```python
from build123d import *

# Parameters (mm, degrees)
SKETCH5_W                 = 81.2
SKETCH5_H                 = 81.2
BOSS_EXTRUDE3_DEPTH       = 2
SKETCH9_W                 = 81.2
SKETCH9_H                 = 81.2
SKETCH9_W_2               = 75.5
SKETCH9_H_2               = 75.5
BOSS_EXTRUDE5_DEPTH       = 5
SKETCH6_W                 = 42.5
SKETCH6_H                 = 57.5
SKETCH6_W_2               = 38.5
SKETCH6_H_2               = 53.5
BOSS_EXTRUDE4_DEPTH       = 17.4
SKETCH7_W                 = 28.5
SKETCH7_H                 = 43.5
SKETCH7_W_2               = 27
SKETCH7_H_2               = 6
SKETCH7_W_3               = 53
CUT_EXTRUDE1_DEPTH        = 2
SKETCH10_W                = 6.5
SKETCH10_H                = 0.85
BOSS_EXTRUDE6_DEPTH       = 15
BOSS_EXTRUDE7_OUTLINE_W   = 81.2
BOSS_EXTRUDE7_OUTLINE_H   = 81.2
BOSS_EXTRUDE7_OUTLINE_W_2 = 79.2
BOSS_EXTRUDE7_OUTLINE_H_2 = 79.2
BOSS_EXTRUDE7_OUTLINE_W_3 = 77.5
BOSS_EXTRUDE7_OUTLINE_H_3 = 77.5
BOSS_EXTRUDE7_OUTLINE_W_4 = 75.5
BOSS_EXTRUDE7_OUTLINE_H_4 = 75.5
BOSS_EXTRUDE7_DEPTH       = 5


# Read off the part's stored shape, not the designer's step: Boss-Extrude7
with BuildPart() as part:
    # Sketch5 → Boss-Extrude3 (new body)
    with BuildSketch(Plane(origin=(0, 0, 0), x_dir=(1, 0, 0), z_dir=(0, 1, 0))):
        with Locations((39.6, 39.6)):
            Rectangle(SKETCH5_W, SKETCH5_H)
    extrude(amount=BOSS_EXTRUDE3_DEPTH)

    # Sketch9 → Boss-Extrude5 (add)
    with BuildSketch(Plane.XZ):
        with Locations((39.6, -39.6)):
            Rectangle(SKETCH9_W, SKETCH9_H)
        with Locations((39.6, -39.6)):
            Rectangle(SKETCH9_W_2, SKETCH9_H_2, mode=Mode.SUBTRACT)
    extrude(amount=BOSS_EXTRUDE5_DEPTH)

    # Sketch6 → Boss-Extrude4 (add)
    with BuildSketch(Plane.XZ):
        with Locations((52.1, -39.6)):
            Rectangle(SKETCH6_W, SKETCH6_H)
        with Locations((52.1, -39.6)):
            Rectangle(SKETCH6_W_2, SKETCH6_H_2, mode=Mode.SUBTRACT)
    extrude(amount=BOSS_EXTRUDE4_DEPTH)

    # Sketch7 → Cut-Extrude1 (cut)
    with BuildSketch(Plane.XZ):
        with Locations((52.1, -39.6)):
            Rectangle(SKETCH7_W, SKETCH7_H)
        with Locations((63.85, -5.85)):
            Rectangle(SKETCH7_W_2, SKETCH7_H_2)
        with Locations((50.85, -73.35)):
            Rectangle(SKETCH7_W_3, SKETCH7_H_2)
    extrude(amount=-CUT_EXTRUDE1_DEPTH, mode=Mode.SUBTRACT)

    # Sketch10 → Boss-Extrude6 (add)
    with BuildSketch(Plane.XZ.offset(5)):
        with Locations((24.5, -0.425)):
            Rectangle(SKETCH10_W, SKETCH10_H)
    extrude(amount=BOSS_EXTRUDE6_DEPTH)

    # Boss-Extrude7 outline → Boss-Extrude7 (add)
    # profile 1 of 2: a face of its own
    with BuildSketch(Plane(origin=(0, -5, 0), x_dir=(-1, 0, 0), z_dir=(0, -1, 0))):
        with Locations((-39.6, 39.6)):
            Rectangle(BOSS_EXTRUDE7_OUTLINE_W, BOSS_EXTRUDE7_OUTLINE_H)
        with Locations((-39.6, 39.6)):
            Rectangle(BOSS_EXTRUDE7_OUTLINE_W_2, BOSS_EXTRUDE7_OUTLINE_H_2, mode=Mode.SUBTRACT)
    # profile 2 of 2: a face of its own
    with BuildSketch(Plane(origin=(0, -5, 0), x_dir=(-1, 0, 0), z_dir=(0, -1, 0))):
        with Locations((-39.6, 39.6)):
            Rectangle(BOSS_EXTRUDE7_OUTLINE_W_3, BOSS_EXTRUDE7_OUTLINE_H_3)
        with Locations((-39.6, 39.6)):
            Rectangle(BOSS_EXTRUDE7_OUTLINE_W_4, BOSS_EXTRUDE7_OUTLINE_H_4, mode=Mode.SUBTRACT)
    extrude(amount=BOSS_EXTRUDE7_DEPTH)


solid = part.part
```
Here's how the part is built. I have some questions about the finished solid (model axes, mm). A direction names the side the tool comes from. Give positions to 0.01 mm unless a question says otherwise; leave off trailing zeros. Write each loop counter-clockwise with the first axis right and the second up, starting at its lowest first coordinate (ties: lowest second). Pieces come first, ordered by that corner, then holes. Notation, with made-up numbers: (57, 0) -> (106, 0) arc R26 ccw to (106, 29) -> close; hole circle Ø1 at (85.25, 20). An arc over 180 degrees is marked (long way). Use one line per item in the form item = value.
1) If I drill on L1, parallel to X at y = -8, z = -65; L2, parallel to X at y = -8.5, z = -10; L3, parallel to Z at x = 67, y = 0.25, over which ranges is the centre line in solid material (lowest first)? Write a range as [from, to].
Verdict:
L1 = [-1, 0], [0.85, 1.85], [30.85, 32.85], [71.35, 73.35], [77.35, 78.35], [79.2, 80.2]
L2 = [-1, 0], [0.85, 1.85], [77.35, 78.35], [79.2, 80.2]
L3 = [-80.2, -76.35], [-70.35, -8.85], [-2.85, 1]
2) I'm going to push flat-ended pins straight in: pin 1 (8 mm diameter, centred on x = 61.5, z = -26, fed in from +Y); pin 2 (8 mm diameter, centred on x = 53, y = -15.5, fed in from +Z); pin 3 (12.5 mm diameter, centred on x = 62, z = -47.5, fed in from -Y); pin 4 (5 mm diameter, centred on x = 46.5, y = -11, fed in from +Z). Where does each tip first touch, or does it pass through?
Verdict:
pin_1 = through
pin_2 = -10.85
pin_3 = 0
pin_4 = 1
3) On a 3-axis mill with a long thin cutter (end or side, diameter ignored), from which of +Z, -Z, +X, -X, +Y, -Y can I reach the whole of each face in a straight line? I mean faces 1 (the face through (37.85, 1, -40)), 2 (the face through (32, -17.4, -39)), 3 (the face through (52, -9, -12.85)). Say none if no direction works.
Verdict:
face_1 = +Y, -Y
face_2 = +Z, -Z, +X, -X, -Y
face_3 = -Y
4) Suppose I cut it at C-C (y = -3). Please give me the cut outline in (x, z), and give its area (3 significant figures).
Verdict:
outline = (-1, -80.2) -> (80.2, -80.2) -> (80.2, 1) -> (-1, 1) -> close; (30.85, -68.35) -> (73.35, -68.35) -> (73.35, -10.85) -> (30.85, -10.85) -> close; hole (1.85, -77.35) -> (77.35, -77.35) -> (77.35, -1.85) -> (1.85, -1.85) -> close; hole (32.85, -66.35) -> (71.35, -66.35) -> (71.35, -12.85) -> (32.85, -12.85) -> close
area = 1,280 mm2
5) Suppose I cut it at B-B (z = -73). Please give me the cut outline in (x, y), and give its area (3 significant figures).
Verdict:
outline = (-1, -10) -> (0, -10) -> (0, -5) -> (0.85, -5) -> (0.85, -10) -> (1.85, -10) -> (1.85, 0) -> (24.35, 0) -> (24.35, 2) -> (-1, 2) -> close; (77.35, -10) -> (78.35, -10) -> (78.35, -5) -> (79.2, -5) -> (79.2, -10) -> (80.2, -10) -> (80.2, 2) -> (77.35, 2) -> close
area = 105 mm2
6) Suppose I cut it at D-D (x = 48). Give the number of separate pieces and of enclosed holes in the cut face, and give its area (4 significant figures).
Verdict:
separate_pieces = 3
enclosed_holes = 0
area = 181.5 mm2
7) We'd pull the mould along X, two halves only. Please class faces 4 (the face through (24, -15, 0)), 5 (the face through (52, -9, -10.85)): +X half, -X half, draft (parallel to the pull), parting line (faces both ways), or undercut.
Verdict:
face_4 = draft
face_5 = undercut
8) Suppose I cut it at A-A (y = -9). Please give me the cut outline in (x, z), and give its area (3 significant figures).
Verdict:
outline = (-1, -80.2) -> (80.2, -80.2) -> (80.2, 1) -> (-1, 1) -> close; (30.85, -68.35) -> (73.35, -68.35) -> (73.35, -10.85) -> (30.85, -10.85) -> close; hole (0, -79.2) -> (79.2, -79.2) -> (79.2, 0) -> (27.75, 0) -> (27.75, -0.85) -> (78.35, -0.85) -> (78.35, -78.35) -> (0.85, -78.35) -> (0.85, -0.85) -> (21.25, -0.85) -> (21.25, 0) -> (0, 0) -> close; hole (1.85, -77.35) -> (77.35, -77.35) -> (77.35, -1.85) -> (1.85, -1.85) -> close; hole (32.85, -66.35) -> (71.35, -66.35) -> (71.35, -12.85) -> (32.85, -12.85) -> close
area = 1,020 mm2
